Model file for the job. Use its own axes, mm. Face numbers are marked on the shaded views. A direction names the side the tool comes from. Give positions to 0.01 mm unless a question says otherwise; leave off trailing zeros. Order: outer loops, then holes, each group sorted by start corner. A loop starts at its lowest first (then second) coordinate and runs counter-clockwise, first axis right, second up. Notation, with made-up numbers: M 72,23 L 83,23 A8 cw 83,36 Z; hole C 65.5,23 d5. An arc over 180 degrees is marked long. Return JSON: item names as keys, results as strings. Group by question number.
1. Wall check: probe 1 along Z at (x, y) = (-4, 8.4); probe 2 along Z at (x, y) = (5, 5); probe 3 along X at (y, z) = (3, -0.25). Give the ranges that are in metal, low to high. Write a range as [from, to].
2. 3-axis set-ups, long thin cutter, end or side, ignore diameter. For the marked faces 4, 5 and 6: which of +Z, -Z, +X, -X, +Y, -Y reach the whole face in a straight line?
3. Two-plate mould, pull along X, no slides. Class the marked faces 1, 2 and 3: released by +X, released by -X, zero draft, split by the parting line, or undercut.
4. Pin check, flat tips, straight feed: pin 1 (6 mm diameter, centred on x = 0, z = 0, fed in from +Y); pin 2 (0.5 mm diameter, centred on x = -4, z = 4, fed in from -Y); pin 3 (1.8 mm diameter, centred on x = 4, z = -4, fed in from -Y). Stop position of each tip, or through.
5. Slice it at C-C on y = 8.75. List the corners of the cut face in (x, z).
6. Slice it at A-A on y = 2. List the corners of the cut face in (x, z) (3 decimals).
7. Slice it at B-B on x = 0. List the corners of the cut face in (y, z) (3 decimals), then the cut area to 3 significant figures.
8. Slice it at D-D on z = 0. List the corners of the cut face in (x, y) (3 decimals), then the cut area to 3 significant figures.
from build123d import *

# Parameters (mm, degrees)
SKETCH_1_W      = 16
SKETCH_1_H      = 16
HEIGHT_DEPTH    = 9.6
SKETCH_2_R      = 2.4
EXTRUDE_2_DEPTH = 1.7
SHELL_1_T       = -1.6
SKETCH_3_R      = 3.255
SKETCH_3_R_2    = 2.4
EXTRUDE_3_DEPTH = 8


with BuildPart() as part:
    # 草圖1 → height (new body)
    with BuildSketch(Plane(origin=(0, 0, 0), x_dir=(1, 0, 0), z_dir=(0, 1, 0))):
        Rectangle(SKETCH_1_W, SKETCH_1_H)
    extrude(amount=HEIGHT_DEPTH)

    # 草圖2 → 填料-伸長2 (add)
    with BuildSketch(Plane(origin=(0, 9.6, 0), x_dir=(1, 0, 0), z_dir=(0, 1, 0))):
        with Locations((-4, 4)):
            Circle(SKETCH_2_R)
        with Locations((4, 4)):
            Circle(SKETCH_2_R)
        with Locations((4, -4)):
            Circle(SKETCH_2_R)
        with Locations((-4, -4)):
            Circle(SKETCH_2_R)
    extrude(amount=EXTRUDE_2_DEPTH)

    # 薄殼1
    shell_1_openings = [part.faces().sort_by_distance(p)[0] for p in [
        (0, 0, 0),
    ]]
    offset(amount=SHELL_1_T, openings=shell_1_openings, kind=Kind.INTERSECTION)

    # 草圖3 → 填料-伸長3 (add)
    with BuildSketch(Plane.XZ.offset(-8)):
        Circle(SKETCH_3_R)
        Circle(SKETCH_3_R_2, mode=Mode.SUBTRACT)
    extrude(amount=EXTRUDE_3_DEPTH)


solid = part.part
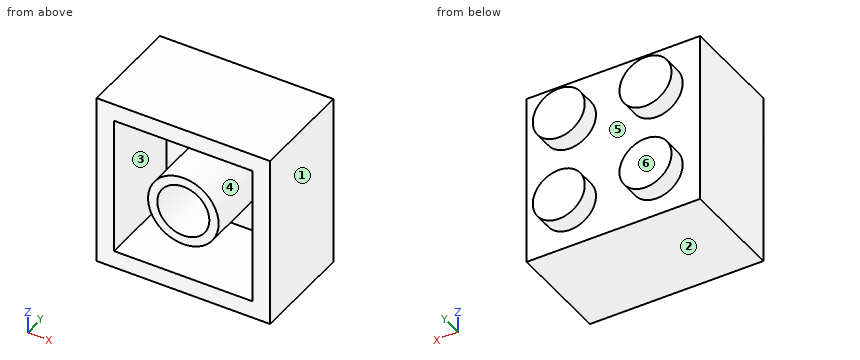
Result:
{
 "1": {"probe 1": "z = [-8, -4.8], [-3.2, 3.2], [4.8, 8]", "probe 2": "z = [-8, -6.4], [6.4, 8]", "probe 3": "x = [-8, -6.4], [-3.25, -2.39], [2.39, 3.25], [6.4, 8]"},
 "2": {"face 4": "-Y", "face 5": "+Y", "face 6": "+Z, -Z, +X, -X, +Y"},
 "3": {"face 1": "released by +X", "face 2": "zero draft", "face 3": "undercut"},
 "4": {"pin 1": "stops at y = 9.6", "pin 2": "stops at y = 9.7", "pin 3": "stops at y = 8"},
 "5": {"outline": "M -8,-8 L 8,-8 L 8,8 L -8,8 Z; hole C -4,-4 d1.6; hole C -4,4 d1.6; hole C 4,-4 d1.6; hole C 4,4 d1.6"},
 "6": {"outline": "M -8,-8 L 8,-8 L 8,8 L -8,8 Z; C 0,0 d6.51; hole M -6.4,-6.4 L 6.4,-6.4 L 6.4,6.4 L -6.4,6.4 Z; hole C 0,0 d4.8"},
 "7": {"outline": "M 0,-8 L 9.6,-8 L 9.6,8 L 0,8 L 0,6.4 L 8,6.4 L 8,3.255 L 0,3.255 L 0,2.4 L 8,2.4 L 8,-2.4 L 0,-2.4 L 0,-3.255 L 8,-3.255 L 8,-6.4 L 0,-6.4 Z", "area": "64.9 mm2"},
 "8": {"outline": "M -8,0 L -6.4,0 L -6.4,8 L -3.255,8 L -3.255,0 L -2.4,0 L -2.4,8 L 2.4,8 L 2.4,0 L 3.255,0 L 3.255,8 L 6.4,8 L 6.4,0 L 8,0 L 8,9.6 L -8,9.6 Z", "area": "64.9 mm2"}
}
